```python
from build123d import *

# Parameters (mm, degrees)
F1_DEPTH = 7.62
F3_D     = 5.08


with BuildPart() as f1:
    # F0 (on Front) → F1 (new body)
    with BuildSketch(Plane.XZ):
        with BuildLine():
            ThreePointArc((53.286768, -21.034017), (9.713758, -19.422437), (-8.682193, 20.109746))
            Line((-8.682193, 20.109746), (-34.082193, 20.109746))
            Line((-34.082193, 20.109746), (-34.082193, 21.38293))
            ThreePointArc((-34.082193, 21.38293), (-3.66046, -41.025575), (65.734673, -43.174696))
            Line((65.734673, -43.174696), (53.286768, -21.034017))
        make_face()
        Polygon((-34.082193, 20.109746), (-8.682193, 20.109746), (-8.682193, 96.309746), (-34.082193, 96.309746), (-34.082193, 21.38293), align=None)
    extrude(amount=F1_DEPTH)

    # F3 (through all)
    with Locations(Plane.XZ.offset(7.62)):
        with Locations((-21.382193, 45.509746)):
            Hole(F3_D / 2)


solid = f1.part
```
Geometry check sheet. Reference: the model listing, model coordinates, mm. A direction names the side the tool comes from. Give positions to 0.01 mm unless a question says otherwise; leave off trailing zeros. Write each loop counter-clockwise with the first axis right and the second up, starting at its lowest first coordinate (ties: lowest second). Pieces come first, ordered by that corner, then holes. Notation, with made-up numbers: (-8, -20) - (19, -20) arc R17 ccw to (19, 6) - close; hole circle Ø7 at (74, -19.5). An arc over 180 degrees is marked (long way). Use a Markdown table: item, result.
Q1. Draft check along Z on faces 1 (the face through (-21, -4, 96.31)), 2 (the face through (-19.37, -3.76, 43.96)), 3 (the face through (-10, -7.62, 6)). Enter one of: pulls with the +Z half, pulls with the -Z half, needs draft (parallel to the pull), parting line crosses it, or undercut.
Computed:
| item | result |
|---|---|
| face 1 | pulls with the +Z half |
| face 2 | undercut |
| face 3 | needs draft |
Q2. Thickness scan on L1, parallel to X at y = -0.25, z = 71; L2, parallel to Z at x = 34, y = -4.25; L3, parallel to X at y = -1.5, z = 15. Record the ranges inside material, lowest first. Write a range as [from, to].
Computed:
| item | result |
|---|---|
| L1 | x = [-34.08, -8.68] |
| L2 | z = [-51.78, -26.38] |
| L3 | x = [-34.35, -8.95] |
Q3. Set-up check for faces 4 (the face through (-10, 0, 6)), 5 (the face through (-8.682, -4, 58)), 6 (the face through (-34.082, -4, 59)): record each of +Z, -Z, +X, -X, +Y, -Y from which the full face is reachable in a straight line by a thin tool's end or side.
Computed:
| item | result |
|---|---|
| face 4 | +Z, -Z, +X, -X, +Y |
| face 5 | +Z, +X, +Y, -Y |
| face 6 | +Z, -X, +Y, -Y |
Q4. Go/stop test with flat-tipped pins: P1, Ø3, axis at y = -4, z = -36.5, coming from the -X side; P2, Ø4.5, axis at x = -21.38, z = 45.51, coming from the -Y side; P3, Ø2, axis at x = 24, y = -6, coming from the -Z side; P4, Ø4, axis at y = -2.5, z = -24, coming from the +X side. Record where each tip stops, or that it passes through.
Computed:
| item | result |
|---|---|
| P1 | stops at x = -11.61 |
| P2 | passes through |
| P3 | stops at z = -51.34 |
| P4 | stops at x = 56.08 |
Q5. Section check A-A, the plane y = -5.25. Enter the section's corners in (x, z).
Computed:
| item | result |
|---|---|
| outline | (-34.08, 21.38) arc R67.17 ccw to (65.73, -43.17) - (53.29, -21.03) arc R41.77 cw to (-8.68, 20.11) - (-8.68, 96.31) - (-34.08, 96.31) - close; hole circle Ø5.08 at (-21.38, 45.51) |
Q6. Section check C-C, the plane x = 45.5. Enter the section's corners in (y, z), then the cut area to 3 significant figures.
Computed:
| item | result |
|---|---|
| outline | (-7.62, -50.59) - (0, -50.59) - (0, -24.42) - (-7.62, -24.42) - close |
| area | 199 mm² |
Q7. Section check B-B, the plane z = 63. Enter the section's corners in (x, y).
Computed:
| item | result |
|---|---|
| outline | (-34.08, -7.62) - (-8.68, -7.62) - (-8.68, 0) - (-34.08, 0) - close |
